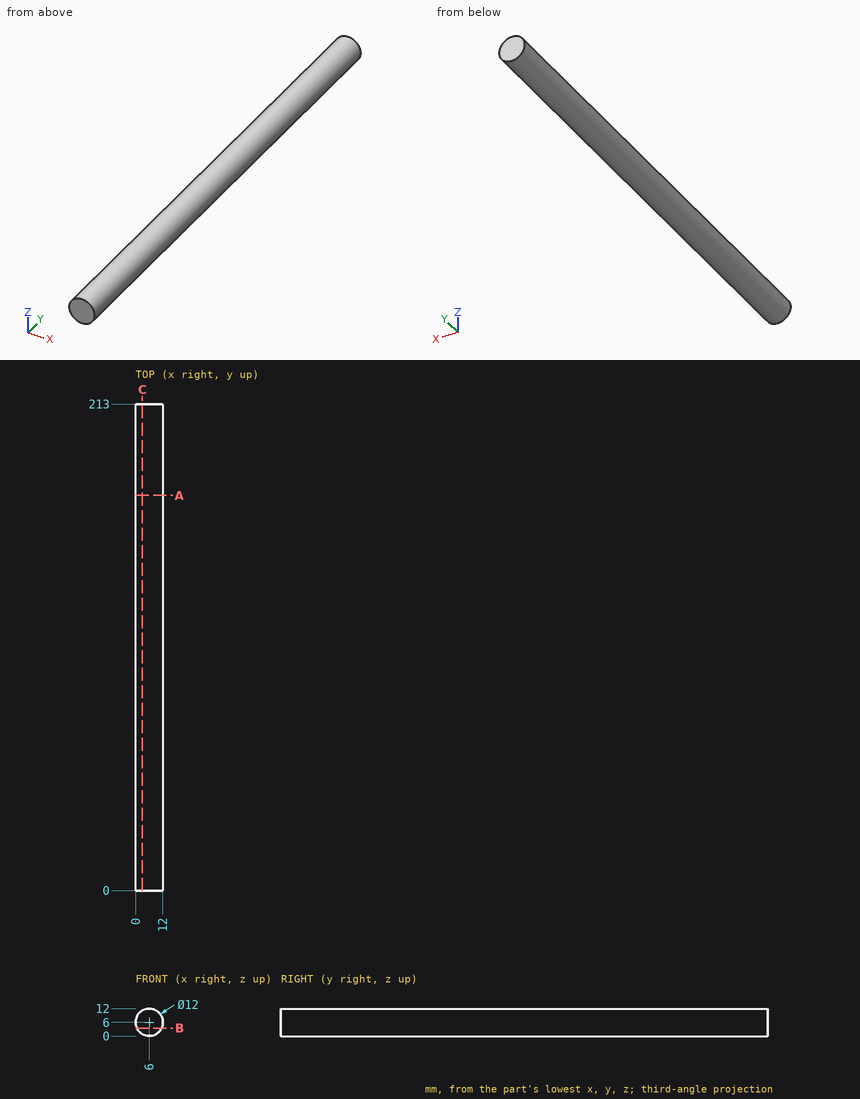
The figure shows three views and two pictorial views of one solid part (mm, origin at its lowest corner). Answer the questions. Round coordinates to 2 decimals unless told otherwise and drop trailing zeros. Write each loop counter-clockwise with the first axis right and the second up, starting at its lowest first coordinate (ties: lowest second). Pieces come first, ordered by that corner, then holes. Notation, with made-up numbers: (20.25, 58.25) -> (35.25, 58.25) arc R18 ccw to (35.25, 92.25) -> close; hole circle Ø4 at (64.25, 86.25). An arc over 180 degrees is marked (long way). Write each question's results on one line, items separated by ' | '.
Q1. Section A-A, the plane y = 173 is taken. Write down the section's boundary in (x, z), then the cut area to 3 significant figures.
Data:
outline: circle Ø12 at (6, 6) | area: 113 mm^2
Q2. Section B-B, the plane z = 3.5 is taken. Write down the section's boundary in (x, y).
Data:
outline: (0.55, 0) -> (11.45, 0) -> (11.45, 213) -> (0.55, 213) -> close
Q3. Straight lines are drawn through the part: line 1 along Z through (x, y) = (2.5, 98); line 2 along X through (y, z) = (202, 0.5); line 3 along Z through (x, y) = (8.75, 101). For each, find the intervals that lie inside material, in ascending order. Write a range as [from, to].
Data:
line 1: [1.13, 10.87] | line 2: [3.6, 8.4] | line 3: [0.67, 11.33]
Q4. Section C-C, the plane x = 3 is taken. Write down the section's boundary in (y, z), then the cut area to 3 significant figures.
Data:
outline: (0, 0.8) -> (213, 0.8) -> (213, 11.2) -> (0, 11.2) -> close | area: 2,210 mm^2
Q5. Flat-ended cylindrical pins translate along their axes: P1, Ø2, axis at y = 105.5, z = 4.5, coming from the +X side; P2, Ø5, axis at x = 9, y = 61.5, coming from the +Z side; P3, Ø1.5, axis at y = 66.5, z = 2, coming from the +X side. Find the tip coordinate at first contact, or state that the pin passes through.
Data:
P1: x = 11.98 | P2: z = 11.98 | P3: x = 11.04
